For this review, take the finished solid that the model builds, in its own axes (mm). Face numbers are marked on the shaded views. A direction names the side the tool comes from. Coordinates: 2 decimals unless noted, no trailing zeros. Order: outer loops, then holes, each group sorted by start corner. A loop starts at its lowest first (then second) coordinate and runs counter-clockwise, first axis right, second up.
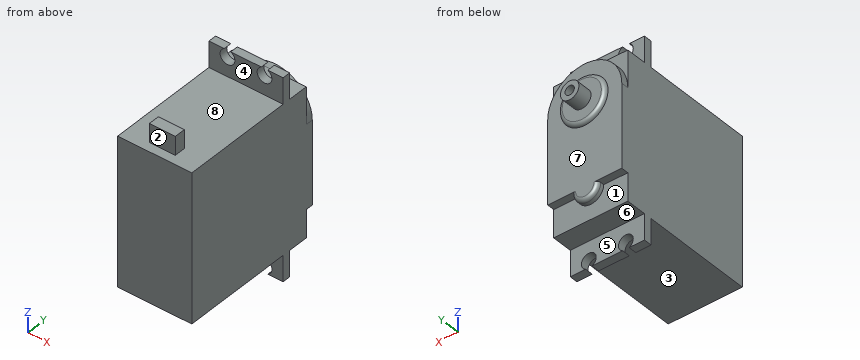
from build123d import *

# Parameters (mm, degrees)
SKETCH1_W                = 20
SKETCH1_H                = 40
BOSS_EXTRUDE1_DEPTH      = 38
SKETCH2_W                = 7
SKETCH2_H                = 3
BOSS_EXTRUDE2_DEPTH      = 5
SKETCH3_R                = 2.5
BOSS_EXTRUDE3_DEPTH      = 7
BOSS_EXTRUDE4_DEPTH      = 7
BOSS_EXTRUDE4_DEPTH_BACK = 47
SKETCH4_W                = 20
SKETCH4_H                = 2.2
SKETCH5_R                = 2
CUT_EXTRUDE1_DEPTH       = 7
BOSS_EXTRUDE5_DEPTH      = 2
SKETCH7_R                = 6.289454611
BOSS_EXTRUDE6_DEPTH      = 1
FILLET1_R                = 1
FILLET2_R                = 1
SKETCH8_R                = 1.25
CUT_EXTRUDE2_DEPTH       = 5


with BuildPart() as part:
    # Sketch1 → Boss-Extrude1 (new body)
    with BuildSketch(Plane(origin=(0, 0, 0), x_dir=(1, 0, 0), z_dir=(0, 1, 0))):
        with Locations((10, 20)):
            Rectangle(SKETCH1_W, SKETCH1_H)
    extrude(amount=BOSS_EXTRUDE1_DEPTH)

    # Sketch2 → Boss-Extrude2 (add)
    with BuildSketch(Plane.XY):
        with Locations((10, 4)):
            Rectangle(SKETCH2_W, SKETCH2_H)
    extrude(amount=BOSS_EXTRUDE2_DEPTH)

    # Sketch3 → Boss-Extrude3 (add)
    with BuildSketch(Plane(origin=(0, 38, 0), x_dir=(1, 0, 0), z_dir=(0, 1, 0))):
        with Locations(Location((10, 10, 0), (0, 0, 90))):
            Circle(SKETCH3_R)
    extrude(amount=BOSS_EXTRUDE3_DEPTH)

    # Sketch4 → Boss-Extrude4 (add, two sides: drawn at the far end of the back side and taken through both)
    with BuildSketch(Plane.XY.offset(-BOSS_EXTRUDE4_DEPTH_BACK)):
        with Locations((10, 31.4)):
            Rectangle(SKETCH4_W, SKETCH4_H)
    extrude(amount=BOSS_EXTRUDE4_DEPTH + BOSS_EXTRUDE4_DEPTH_BACK)

    # Sketch5 → Cut-Extrude1 (cut)
    with BuildSketch(Plane(origin=(0, 32.5, 0), x_dir=(1, 0, 0), z_dir=(0, 1, 0))):
        with Locations((15, 45.2)):
            Circle(SKETCH5_R)
        with Locations((5, 45.2)):
            Circle(SKETCH5_R)
        with Locations((15, -5.2)):
            Circle(SKETCH5_R)
        with Locations((5, -5.2)):
            Circle(SKETCH5_R)
    extrude(amount=-CUT_EXTRUDE1_DEPTH, mode=Mode.SUBTRACT)

    # Sketch6 → Boss-Extrude5 (add)
    with BuildSketch(Plane(origin=(0, 38, 0), x_dir=(1, 0, 0), z_dir=(0, 1, 0))):
        with BuildLine():
            Line((20, 32.5), (13.5, 32.5))
            ThreePointArc((13.5, 32.5), (10, 36), (6.5, 32.5))
            Line((6.5, 32.5), (0, 32.5))
            Line((0, 32.5), (0, 10))
            ThreePointArc((0, 10), (10, 0), (20, 10))
            Line((20, 10), (20, 32.5))
        make_face()
    extrude(amount=BOSS_EXTRUDE5_DEPTH)

    # Sketch7 → Boss-Extrude6 (add)
    with BuildSketch(Plane(origin=(0, 40, 0), x_dir=(1, 0, 0), z_dir=(0, 1, 0))):
        with Locations(Location((10, 10, 0), (0, 0, 270))):
            Circle(SKETCH7_R)
    extrude(amount=BOSS_EXTRUDE6_DEPTH)

    # Fillet1
    fillet1_edges = [part.edges().sort_by_distance(p)[0] for p in [
        (10, 41, -16.289454611),
    ]]
    fillet(fillet1_edges, radius=FILLET1_R - 0.0001)  # a hair under: the kernel refuses the full size

    # Fillet2
    fillet2_edges = [part.edges().sort_by_distance(p)[0] for p in [
        (10, 40, -36),
    ]]
    fillet(fillet2_edges, radius=FILLET2_R)

    # Sketch8 → Cut-Extrude2 (cut)
    with BuildSketch(Plane(origin=(0, 45, 0), x_dir=(1, 0, 0), z_dir=(0, 1, 0))):
        with Locations(Location((10, 10, 0), (0, 0, 270))):
            Circle(SKETCH8_R)
    extrude(amount=-CUT_EXTRUDE2_DEPTH, mode=Mode.SUBTRACT)


solid = part.part
1. Take a section at B-B, the plane z = -42. Give the boundary of the cut face in (x, y).
Answer below:
outline: (0, 30.3) - (20, 30.3) - (20, 32.5) - (0, 32.5) - close
2. To check wall thickness, follow L1, parallel to X at y = 31, z = 5; L2, parallel to X at y = 42.95, z = -10; L3, parallel to Z at x = 16.5, y = 9. State the ranges of each line that lie inside material, in increasing order.
Answer below:
L1: x = 0 to 3.01, 6.99 to 13.01, 16.99 to 20
L2: x = 7.5 to 8.75, 11.25 to 12.5
L3: z = -40 to 0
3. The part is to be moulded in two halves that separate along Y. For the marked faces 6, 7 and 8, say which applies: +Y half, -Y half, draft (parallel to the pull), parting line (faces both ways), or undercut.
Answer below:
face 6: draft
face 7: +Y half
face 8: undercut
4. Machinability: for the marked faces 1, 2, 3, 4 and 5, which of the approach directions +Z, -Z, +X, -X, +Y, -Y give a long, thin tool a straight path to every point of the face, cutting with its end or side? Answer none if there is none.
Answer below:
face 1: -Z, +Y
face 2: +Z, +X, -X, -Y
face 3: -Z, +X, -X, -Y
face 4: +Z, +X, -X
face 5: -Z, +X, -X, +Y
5. Take a section at C-C, the plane x = 17.75. Give the boundary of the cut face in (y, z).
Answer below:
outline: (0, -40) - (30.3, -40) - (30.3, -47) - (32.5, -47) - (32.5, -40) - (38, -40) - (38, -32.5) - (40, -32.5) - (40, -3.68) - (38, -3.68) - (38, 0) - (32.5, 0) - (32.5, 7) - (30.3, 7) - (30.3, 0) - (0, 0) - close
6. Take a section at D-D, the plane y = 19.5. Give the boundary of the cut face in (x, z).
Answer below:
outline: (0, -40) - (20, -40) - (20, 0) - (0, 0) - close
7. Clearance check with flat-ended pins moving along their axes: pin 1 Ø3 at (x, z) = (3, -35.5) entering from +Y; pin 2 Ø1.5 at (y, z) = (4.5, 3) entering from +X; pin 3 Ø3 at (x, z) = (8, -22) entering from +Y; pin 4 Ø2.5 at (x, z) = (15, 5.2) entering from -Y. State where each tip first meets the part, or that it passes through.
Answer below:
pin 1: stops at y = 38
pin 2: stops at x = 13.5
pin 3: stops at y = 40
pin 4: passes through
8. Take a section at A-A, the plane y = 4.5. Give the boundary of the cut face in (x, z), plus the area to 3 significant figures.
Answer below:
outline: (0, -40) - (20, -40) - (20, 0) - (13.5, 0) - (13.5, 5) - (6.5, 5) - (6.5, 0) - (0, 0) - close
area: 835 mm2
